from build123d import *

# Parameters (mm, degrees)
F1_DEPTH = 127
F0_W     = 20.32
F0_H     = 12.833738
F0_H_2   = 10.154468
F2_DEPTH = 120.65
F0_W_2   = 111.76
F0_H_3   = 17.412408
F3_DEPTH = 6.35


with BuildPart() as f1:
    # F0 (on Front) → F1 (new body)
    with BuildSketch(Plane.XZ):
        Polygon((190.410141, 39.868113), (-190.589859, 39.868113), (-190.589859, 27.168113), (-184.239859, 27.168113), (-163.919859, 27.168113), (-62.319859, 27.168113), (-55.969859, 27.168113), (55.790141, 27.168113), (62.140141, 27.168113), (163.740141, 27.168113), (184.060141, 27.168113), (190.410141, 27.168113), align=None)
    extrude(amount=F1_DEPTH)

    # F0 (on Front) → F2 (join)
    with BuildSketch(Plane.XZ):
        with BuildLine():
            Line((-163.919859, -61.731887), (-184.239859, -61.731887))
            Line((-184.239859, -61.731887), (-184.239859, -99.831887))
            Line((-184.239859, -99.831887), (-148.679859, -99.831887))
            add(Edge.make_bspline(
                [(-148.679859, -99.831887), (-148.487159, -86.25736), (-74.288484, -80.346777), (-0.089859, -80.781887)],
                knots=[0, 0, 0, 0, 148.535829, 148.535829, 148.535829, 148.535829], degree=3))
            Line((-0.089859, -80.781887), (-0.089859, -61.731887))
            Line((-0.089859, -61.731887), (-55.969859, -61.731887))
            Line((-55.969859, -61.731887), (-62.319859, -61.731887))
            Line((-62.319859, -61.731887), (-163.919859, -61.731887))
        make_face()
        with BuildLine():
            Line((184.060141, -99.831887), (184.060141, -61.731887))
            Line((184.060141, -61.731887), (163.740141, -61.731887))
            Line((163.740141, -61.731887), (62.140141, -61.731887))
            Line((62.140141, -61.731887), (55.790141, -61.731887))
            Line((55.790141, -61.731887), (-0.089859, -61.731887))
            Line((-0.089859, -61.731887), (-0.089859, -80.781887))
            add(Edge.make_bspline(
                [(-0.089859, -80.781887), (74.162886, -81.217313), (148.41558, -88.007693), (148.500141, -99.831887)],
                knots=[148.535829, 148.535829, 148.535829, 148.535829, 297.18, 297.18, 297.18, 297.18], degree=3))
            Line((148.500141, -99.831887), (184.060141, -99.831887))
        make_face()
        with Locations((173.900141, -55.315018)):
            Rectangle(F0_W, F0_H)
        Polygon((184.060141, -48.898149), (184.060141, 27.168113), (163.740141, 27.168113), (163.740141, -24.726205), (163.740141, -48.898149), align=None)
        Polygon((62.140141, -9.948243), (62.140141, 27.168113), (55.790141, 27.168113), (55.790141, 9.755705), (55.790141, -9.948243), align=None)
        Polygon((62.140141, -24.726205), (62.140141, -9.948243), (55.790141, -9.948243), (55.790141, -61.731887), (62.140141, -61.731887), align=None)
        Polygon((-163.919859, 27.168113), (-184.239859, 27.168113), (-184.239859, -51.577419), (-163.919859, -51.577419), (-163.919859, -26.83734), align=None)
        with Locations((-174.079859, -56.654653)):
            Rectangle(F0_W, F0_H_2)
        Polygon((-55.969859, 27.168113), (-62.319859, 27.168113), (-62.319859, -2.911118), (-55.969859, -2.911118), (-55.969859, 9.755705), align=None)
        Polygon((-55.969859, -2.911118), (-62.319859, -2.911118), (-62.319859, -26.83734), (-62.319859, -61.731887), (-55.969859, -61.731887), align=None)
    extrude(amount=F2_DEPTH)

    # F0 (on Front) → F3 (join)
    with BuildSketch(Plane.XZ):
        Polygon((-62.319859, 27.168113), (-163.919859, 27.168113), (-163.919859, -26.83734), (-62.319859, -26.83734), (-62.319859, -2.911118), align=None)
        Polygon((-163.919859, -26.83734), (-163.919859, -51.577419), (-163.919859, -61.731887), (-62.319859, -61.731887), (-62.319859, -26.83734), align=None)
        with Locations((-0.089859, 18.461909)):
            Rectangle(F0_W_2, F0_H_3)
        Polygon((55.790141, 9.755705), (-55.969859, 9.755705), (-55.969859, -2.911118), (-55.969859, -61.731887), (-0.089859, -61.731887), (55.790141, -61.731887), (55.790141, -9.948243), align=None)
        Polygon((163.740141, -24.726205), (163.740141, 27.168113), (62.140141, 27.168113), (62.140141, -9.948243), (62.140141, -24.726205), align=None)
        Polygon((163.740141, -61.731887), (163.740141, -48.898149), (163.740141, -24.726205), (62.140141, -24.726205), (62.140141, -61.731887), align=None)
    extrude(amount=F3_DEPTH)


solid = f1.part
Model file for the job. Use its own axes, mm. A direction names the side the tool comes from. Give positions to 0.01 mm unless a question says otherwise; leave off trailing zeros. Loops run counter-clockwise (first coordinate to the right, second up) from the corner with the lowest first, then second, coordinate; pieces in that order, holes last. Notation, with made-up numbers: (87.25, -17) -> (104.25, -17) arc R30 ccw to (104.25, 18) -> close; hole circle Ø8 at (47.25, -13). An arc over 180 degrees is marked (long way). Use a Markdown table: item, result. Add a question column.
(1) Slice it at A-A on z = -33.5. List the corners of the cut face in (x, y).
(2) Tool access for faces 4 (the flat face through (-55.97, -63, -18)), 5 (the flat face through (184.06, -59, -37)), 6 (the flat face through (-3, 0, -29)): list every direction of +Z, -Z, +X, -X, +Y, -Y with a clear straight run to the whole face (end or side of a thin tool).
(3) Drop flat-ended pins along their axis: pin 1 Ø2 at (y, z) = (-52.5, 0.5) entering from -X; pin 2 Ø5 at (x, z) = (132.5, -72) entering from -Y; pin 3 Ø8 at (x, z) = (14, -38) entering from -Y. Give the stop position or say it passes through.
(4) Wall check: line 1 along X through (y, z) = (-115.5, -35); line 2 along Y through (x, z) = (-64, -70); line 3 along Z through (x, y) = (-17, -109). Give the ranges that are in metal, low to high.
(5) Slice it at B-B on y = -71. Give the number of separate pieces and of enclosed holes in the cut face, and give its area (3 significant figures).
(6) Mould opens along X. For faces 1 (the flat face through (-114, -6.35, -17)), 2 (the flat face through (-167, -59, -99.832)), 3 (the flat face through (-184.24, -59, -35)) say: +X half, -X half, draft (parallel to the pull), parting line (faces both ways), or undercut.
Filled sheet:
| question | item | result |
|---|---|---|
| 1 | outline | (-184.24, -120.65) -> (-163.92, -120.65) -> (-163.92, -6.35) -> (-62.32, -6.35) -> (-62.32, -120.65) -> (-55.97, -120.65) -> (-55.97, -6.35) -> (55.79, -6.35) -> (55.79, -120.65) -> (62.14, -120.65) -> (62.14, -6.35) -> (163.74, -6.35) -> (163.74, -120.65) -> (184.06, -120.65) -> (184.06, 0) -> (-184.24, 0) -> close |
| 2 | face 4 | -Y |
| 2 | face 5 | -Z, +X, +Y, -Y |
| 2 | face 6 | +Z, -Z, +X, -X, +Y |
| 3 | pin 1 | x = -184.24 |
| 3 | pin 2 | y = -120.65 |
| 3 | pin 3 | y = -6.35 |
| 4 | line 1 | -184.24 to -163.92, -62.32 to -55.97, 55.79 to 62.14, 163.74 to 184.06 |
| 4 | line 2 | -120.65 to 0 |
| 4 | line 3 | -80.79 to -61.73, 27.17 to 39.87 |
| 5 | separate pieces | 1 |
| 5 | enclosed holes | 3 |
| 5 | area | 19,100 mm2 |
| 6 | face 1 | undercut |
| 6 | face 2 | draft |
| 6 | face 3 | -X half |
